The listing builds one solid part. Answer for the finished solid, in the listing's coordinates (mm). A direction names the side the tool comes from. Give positions to 0.01 mm unless a question says otherwise; leave off trailing zeros. Loops run counter-clockwise (first coordinate to the right, second up) from the corner with the lowest first, then second, coordinate; pieces in that order, holes last. Notation, with made-up numbers: (53.5, 31.25) - (59.5, 31.25) arc R30 cw to (59.5, 63.25) - close; hole circle Ø1 at (47.25, 5.25). An arc over 180 degrees is marked (long way). Write item = value, one per line. Start each with the question number.
1) The part is cut by section A-A on x = -14. Write down the section's boundary in (y, z), plus the area to 4 significant figures.
2) Consider probe 1 along Y at (x, z) = (19, 4.8); probe 2 along Y at (x, z) = (-2, 2.4); probe 3 along Y at (x, z) = (0, 3.35). Determine where each line is inside the solid, lowest interval first.
3) Flat-ended cylindrical pins translate along their axes: P1, Ø5.5, axis at x = -14, y = 7, coming from the -Z side; P2, Ø2, axis at y = -13, z = 2.5, coming from the -X side; P3, Ø1.2, axis at x = -22, z = 2.5, coming from the -Y side; P4, Ø1.5, axis at x = 19.5, z = 1.5, coming from the -Y side. Find the tip coordinate at first contact, or state that the pin passes through.
4) The mould has two halves that part along Y. Classify faces 4 (the flat face through (26, -24, 2)), 5 (the flat face through (-19.2, -23, 2)), 6 (the flat face through (-19.2, -7, 2)): +Y half, -Y half, draft (parallel to the pull), parting line (faces both ways), or undercut.
5) The part is cut by section B-B on x = -2. Write down the section's boundary in (y, z).
6) Which of the six approach directions +Z, -Z, +X, -X, +Y, -Y give full straight-line access (tool end or side, diameter ignored) to faces 1 (the flat face through (-20, 9, 2)), 2 (the flat face through (21, -1.5, 2)), 3 (the flat face through (32, -5, 0))?
7) The part is cut by section C-C on z = 3.15. State how many separate pieces and enclosed holes the cut face has, plus the area to 3 significant figures.
from build123d import *

# Parameters (mm, degrees)
SKETCH1_R           = 5.98
SKETCH1_R_2         = 1.65
SKETCH1_W           = 9
SKETCH1_H           = 5
SKETCH1_H_2         = 3
SKETCH1_W_2         = 7.5
SKETCH1_H_3         = 6
BOSS_EXTRUDE1_DEPTH = 5
FILLET1_R           = 1.2
FILLET2_R           = 3
FILLET3_R           = 1
FILLET5_R           = 1.8
FILLET6_R           = 0.8
FILLET7_R           = 3


with BuildPart() as part:
    # Sketch1 → Boss-Extrude1 (new body)
    with BuildSketch(Plane.XY):
        with BuildLine():
            Line((72.356568311, -24), (75.172081726, -33))
            Line((75.172081726, -33), (80.827918274, -33))
            Line((80.827918274, -33), (88.70873293, -17.415075165))
            ThreePointArc((88.70873293, -17.415075165), (89.67272023, -14.78345153), (90, -12))
            Line((90, -12), (90, -4))
            ThreePointArc((90, -4), (86.485281374, 4.485281374), (78, 8))
            Line((78, 8), (28, 8))
            Line((28, 8), (28, 12))
            Line((28, 12), (-20, 12))
            Line((-20, 12), (-20, 6.6))
            ThreePointArc((-20, 6.6), (-19.2, 5.8), (-20, 5))
            Line((-20, 5), (-22, 5))
            Line((-22, 5), (-22, 2))
            Line((-22, 2), (-19.449413077, -0.419608718))
            ThreePointArc((-19.449413077, -0.419608718), (-19.264993354, -0.684143655), (-19.2, -1))
            Line((-19.2, -1), (-19.2, -13))
            ThreePointArc((-19.2, -13), (-20.078679656, -15.121320344), (-22.2, -16))
            Line((-22.2, -16), (-25, -16))
            Line((-25, -16), (-25, -21))
            Line((-25, -21), (-23, -22.5))
            Line((-23, -22.5), (-21.5, -22.5))
            Line((-21.5, -22.5), (-21.5, -21.5))
            ThreePointArc((-21.5, -21.5), (-21.353553391, -21.146446609), (-21, -21))
            Line((-21, -21), (-20, -21))
            ThreePointArc((-20, -21), (-19.434314575, -21.234314575), (-19.2, -21.8))
            Line((-19.2, -21.8), (-19.2, -24))
            Line((-19.2, -24), (72.356568311, -24))
        make_face()
        Circle(SKETCH1_R, mode=Mode.SUBTRACT)
        with Locations((78, -12)):
            Circle(SKETCH1_R, mode=Mode.SUBTRACT)
        with Locations((-14, 7)):
            Circle(SKETCH1_R_2, mode=Mode.SUBTRACT)
        with Locations((-2, -18)):
            Circle(SKETCH1_R_2, mode=Mode.SUBTRACT)
        with Locations((21, -13.5)):
            Rectangle(SKETCH1_W, SKETCH1_H, mode=Mode.SUBTRACT)
        with Locations((21, -3)):
            Rectangle(SKETCH1_W, SKETCH1_H_2, mode=Mode.SUBTRACT)
        with Locations((11.25, -11)):
            Rectangle(SKETCH1_W_2, SKETCH1_H_3, mode=Mode.SUBTRACT)
    extrude(amount=BOSS_EXTRUDE1_DEPTH)

    # Fillet1
    fillet1_edges = [part.edges().sort_by_distance(p)[0] for p in [
        (16.5, -11, 2.5),
        (16.5, -16, 2.5),
        (25.5, -16, 2.5),
        (25.5, -11, 2.5),
        (16.5, -1.5, 2.5),
        (16.5, -4.5, 2.5),
        (25.5, -4.5, 2.5),
        (25.5, -1.5, 2.5),
    ]]
    fillet(fillet1_edges, radius=FILLET1_R)

    # Fillet2
    fillet2_edges = [part.edges().sort_by_distance(p)[0] for p in [
        (28, 8, 2.5),
    ]]
    fillet(fillet2_edges, radius=FILLET2_R)

    # Fillet3
    fillet3_edges = [part.edges().sort_by_distance(p)[0] for p in [
        (28, 12, 2.5),
        (-20, 12, 2.5),
    ]]
    fillet(fillet3_edges, radius=FILLET3_R - 0.0001)  # a hair under: the kernel refuses the full size

    # Fillet5
    fillet5_edges = [part.edges().sort_by_distance(p)[0] for p in [
        (7.5, -8, 2.5),
        (7.5, -14, 2.5),
        (15, -14, 2.5),
        (15, -8, 2.5),
    ]]
    fillet(fillet5_edges, radius=FILLET5_R)

    # Fillet6
    fillet6_edges = [part.edges().sort_by_distance(p)[0] for p in [
        (-22, 5, 2.5),
    ]]
    fillet(fillet6_edges, radius=FILLET6_R)

    # Fillet7
    fillet7_edges = [part.edges().sort_by_distance(p)[0] for p in [
        (-25, -16, 2.5),
    ]]
    fillet(fillet7_edges, radius=FILLET7_R)


solid = part.part
Answer below:
q1.outline = (-24, 0) - (5.35, 0) - (5.35, 5) - (-24, 5) - close; (8.65, 0) - (12, 0) - (12, 5) - (8.65, 5) - close
q1.area = 163.5 mm2
q2.probe_1 = -24 to -16, -11 to -4.5, -1.5 to 12
q2.probe_2 = -24 to -19.65, -16.35 to -5.64, 5.64 to 12
q2.probe_3 = -24 to -5.98, 5.98 to 12
q3.P1 = 0
q3.P2 = -19.37
q3.P3 = -22.5
q3.P4 = -24
q4.face_4 = -Y half
q4.face_5 = draft
q4.face_6 = undercut
q5.outline = (-24, 0) - (-19.65, 0) - (-19.65, 5) - (-24, 5) - close; (-16.35, 0) - (-5.64, 0) - (-5.64, 5) - (-16.35, 5) - close; (5.64, 0) - (12, 0) - (12, 5) - (5.64, 5) - close
q6.face_1 = +Z, -Z, -X, +Y
q6.face_2 = +Z, -Z
q6.face_3 = -Z, +X, -X, +Y, -Y
q7.separate_pieces = 1
q7.enclosed_holes = 7
q7.area = 3,410 mm2
